```python
from build123d import *

# Parameters (mm, degrees)
SKETCH079_R           = 62.5
SKETCH079_R_2         = 47.5
PAD055_DEPTH          = 1.6
SKETCH080_W           = 4
SKETCH080_H           = 8
PAD056_DEPTH          = 1.5
POLARPATTERN011_COUNT = 20


with BuildPart() as part:
    # Sketch079 → Pad055 (new body)
    with BuildSketch(Plane.XY):
        Circle(SKETCH079_R)
        Circle(SKETCH079_R_2, mode=Mode.SUBTRACT)
    extrude(amount=PAD055_DEPTH)

    # Sketch080 (on Face3 of Pad055) → Pad056 (join)
    with BuildSketch(Plane(origin=(0, 0, 0), x_dir=(1, 0, 0), z_dir=(0, 0, -1))):
        with Locations((-55, 0)):
            Rectangle(SKETCH080_W, SKETCH080_H)
    pad056 = extrude(amount=PAD056_DEPTH)

    # PolarPattern011: Pad056 ×20 about axis
    polarpattern011_axis = Axis((0, 0, 0), (0, 0, -1))
    for i in range(1, POLARPATTERN011_COUNT):
        add(pad056.rotate(polarpattern011_axis, i * 360 / POLARPATTERN011_COUNT))


with BuildPart() as part_1:
    # Body032 placement: moved
    add(part.part.moved(Location((0, 0, 2))))


solid = part_1.part
```
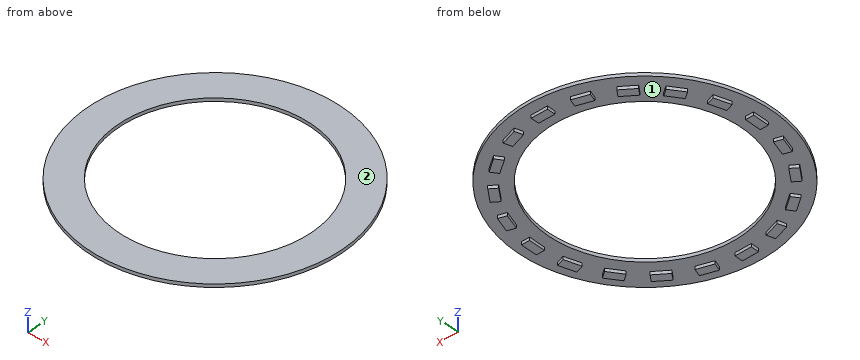
The model under review builds one solid part; all positions refer to its coordinate system, in mm. Face numbers are marked on the shaded views. Round coordinates to 2 decimals unless told otherwise and drop trailing zeros. Write each loop counter-clockwise with the first axis right and the second up, starting at its lowest first coordinate (ties: lowest second). Pieces come first, ordered by that corner, then holes. Notation, with made-up numbers: M 51.5,10.5 L 86.5,10.5 A17 cw 86.5,41.5 Z; hole C -10.75,-37.75 d4. An arc over 180 degrees is marked long. Use CSV: the item, a comma, the result in double quotes. Start each with the question number.
(1) The part is to be moulded in two halves that separate along Y. For the marked faces 1 and 2, say which applies: +Y half, -Y half, draft (parallel to the pull), parting line (faces both ways), or undercut.
(2) For line 1 along Y through (x, z) = (-2.5, 1.6); line 2 along Y through (x, z) = (0, 2.75); line 3 along X through (y, z) = (31, 3.1), list the stretches that pass through material, from the lowest coordinate up.
(3) We need section D-D, the plane y = -23. State the section outline as (x, z) points.
(4) We need section A-A, the plane x = 0. State the section outline as (y, z) points, then the cut area to 3 significant figures.
(5) We need section C-C, the plane z = 2.8. State the section outline as (x, y) points, then the cut area to 3 significant figures.
(6) Clearance check with flat-ended pins moving along their axes: P1, Ø1.6, axis at x = 55, z = 1.5, coming from the -Y side; P2, Ø1.6, axis at y = 1.5, z = 1, coming from the -X side; P3, Ø1.6, axis at x = -55.5, z = 1.5, coming from the -Y side. State where each tip first meets the part, or that it passes through.
Findings:
1,face 1,"undercut"
1,face 2,"draft"
2,line 1,"-57 to -53, 53 to 57"
2,line 2,"-62.5 to -47.5, 47.5 to 62.5"
2,line 3,"-54.27 to -35.99, 35.99 to 54.27"
3,outline,"M -58.11,2 L -41.56,2 L -41.56,3.6 L -58.11,3.6 Z; M 41.56,2 L 58.11,2 L 58.11,3.6 L 41.56,3.6 Z"
4,outline,"M -62.5,2 L -57,2 L -57,0.5 L -53,0.5 L -53,2 L -47.5,2 L -47.5,3.6 L -62.5,3.6 Z; M 47.5,2 L 53,2 L 53,0.5 L 57,0.5 L 57,2 L 62.5,2 L 62.5,3.6 L 47.5,3.6 Z"
4,area,"60.0 mm^2"
5,outline,"C 0,0 d125; hole C 0,0 d95"
5,area,"5,180 mm^2"
6,P1,"y = -30.81"
6,P2,"x = -57"
6,P3,"y = -29.92"
